For this review, take the finished solid that the model builds, in its own axes (mm). A direction names the side the tool comes from. Give positions to 0.01 mm unless a question says otherwise; leave off trailing zeros. Write each loop counter-clockwise with the first axis right and the second up, starting at its lowest first coordinate (ties: lowest second). Pieces come first, ordered by that corner, then holes. Notation, with made-up numbers: (7.25, 45.5) -> (11.25, 45.5) arc R18 ccw to (11.25, 57.5) -> close; hole circle Ø10 at (76, 66). An arc over 180 degrees is marked (long way). Return JSON: item names as keys, results as strings.
from build123d import *

# Parameters (mm, degrees)
SKIZZE1_W                                            = 40
SKIZZE1_H                                            = 7
AUFSATZ_LINEAR_AUSTRAGEN1_DEPTH                      = 35
SKIZZE2_W                                            = 12
SKIZZE2_H                                            = 6.1
SKIZZE2_R                                            = 0.6
AUFSATZ_LINEAR_AUSTRAGEN2_DEPTH                      = 14
FORMSENKUNG_F_R_M3_SENKSCHRAUBE_MIT_SCHL_D           = 3.4
FORMSENKUNG_F_R_M3_SENKSCHRAUBE_MIT_SCHL_CSINK_D     = 6.3
FORMSENKUNG_F_R_M3_SENKSCHRAUBE_MIT_SCHL_CSINK_ANGLE = 90
VERRUNDUNG1_R                                        = 3.5
SCHNITT_LINEAR_AUSTRAGEN1_DEPTH                      = 45.648628198
SCHNITT_LINEAR_AUSTRAGEN2_DEPTH                      = 2


with BuildPart() as part:
    # Skizze1 → Aufsatz-Linear austragen1 (new body)
    with BuildSketch(Plane(origin=(0, 0, 0), x_dir=(1, 0, 0), z_dir=(0, 1, 0))):
        with Locations((1.5, 0)):
            Rectangle(SKIZZE1_W, SKIZZE1_H)
    extrude(amount=AUFSATZ_LINEAR_AUSTRAGEN1_DEPTH)

    # Skizze2 → Aufsatz-Linear austragen2 (add)
    # profile 1 of 2: a face of its own
    with BuildSketch(Plane(origin=(0, 0, -3.5), x_dir=(-1, 0, 0), z_dir=(0, 0, -1))):
        with Locations((-15.5, 31.95)):
            Rectangle(SKIZZE2_W, SKIZZE2_H)
        with Locations((-15.5, 31.75)):
            Circle(SKIZZE2_R, mode=Mode.SUBTRACT)
    # profile 2 of 2: a face of its own
    with BuildSketch(Plane(origin=(0, 0, -3.5), x_dir=(-1, 0, 0), z_dir=(0, 0, -1))):
        with Locations((-15.5, 3.05)):
            Rectangle(SKIZZE2_W, SKIZZE2_H)
        with Locations((-15.5, 3.25)):
            Circle(SKIZZE2_R, mode=Mode.SUBTRACT)
    extrude(amount=AUFSATZ_LINEAR_AUSTRAGEN2_DEPTH)

    # Formsenkung für M3 Senkschraube mit Schlitz/Kreuzschlitz1 (through all)
    with Locations(Plane(origin=(0, 0, -3.5), x_dir=(-1, 0, 0), z_dir=(0, 0, -1))):
        with Locations((-5, 20), (5, 20), (5, 5), (-5, 5)):
            CounterSinkHole(FORMSENKUNG_F_R_M3_SENKSCHRAUBE_MIT_SCHL_D / 2, FORMSENKUNG_F_R_M3_SENKSCHRAUBE_MIT_SCHL_CSINK_D / 2, counter_sink_angle=FORMSENKUNG_F_R_M3_SENKSCHRAUBE_MIT_SCHL_CSINK_ANGLE)

    # Verrundung1
    verrundung1_edges = [part.edges().sort_by_distance(p)[0] for p in [
        (21.5, 17.5, 3.5),
        (-18.5, 17.5, 3.5),
        (-18.5, 17.5, -3.5),
    ]]
    fillet(verrundung1_edges, radius=VERRUNDUNG1_R - 0.0001)  # a hair under: the kernel refuses the full size

    # Skizze1<5> → Schnitt-Linear austragen1 (cut, through all)
    with BuildSketch(Plane(origin=(0, 0, 0), x_dir=(1, 0, 0), z_dir=(0, 1, 0))):
        with BuildLine():
            ThreePointArc((13.45, 0), (15, -1.55), (16.55, 0))
            Line((16.55, 0), (13.45, 0))
        make_face()
        with BuildLine():
            Line((13.45, 0), (16.55, 0))
            ThreePointArc((16.55, 0), (15, 1.55), (13.45, 0))
        make_face()
        with BuildLine():
            ThreePointArc((-16.55, 0), (-15, -1.55), (-13.45, 0))
            Line((-13.45, 0), (-16.55, 0))
        make_face()
        with BuildLine():
            Line((-16.55, 0), (-13.45, 0))
            ThreePointArc((-13.45, 0), (-15, 1.55), (-16.55, 0))
        make_face()
    extrude(amount=SCHNITT_LINEAR_AUSTRAGEN1_DEPTH, mode=Mode.SUBTRACT)

    # Skizze1<7> → Schnitt-Linear austragen2 (cut)
    with BuildSketch(Plane(origin=(0, 0, 0), x_dir=(1, 0, 0), z_dir=(0, 1, 0))):
        with BuildLine():
            ThreePointArc((-2.4, 0), (0, -2.4), (2.4, 0))
            Line((2.4, 0), (-2.4, 0))
        make_face()
        with BuildLine():
            Line((-2.4, 0), (2.4, 0))
            ThreePointArc((2.4, 0), (0, 2.4), (-2.4, 0))
        make_face()
    extrude(amount=SCHNITT_LINEAR_AUSTRAGEN2_DEPTH, mode=Mode.SUBTRACT)


solid = part.part
1. Add section A-A, the plane y = 20. Count the separate pieces of the cut face and the enclosed holes in it, plus the area to 3 significant figures.
Results found:
{"separate pieces": "3", "enclosed holes": "2", "area": "205 mm²"}
2. The part is to be moulded in two halves that separate along Z. For faces 1 (the cylindrical face through (13.45, 17.26, -0.07)), 2 (the cylindrical face through (5.8, 3.5, 0.8)), 3 (the cylindrical face through (-17.5, 17.74, 2.45)), 4 (the flat face through (15.5, 3.2, -3.5)), say which applies: +Z half, -Z half, draft (parallel to the pull), parting line (faces both ways), or undercut.
Results found:
{"face 1": "undercut", "face 2": "draft", "face 3": "+Z half", "face 4": "-Z half"}
3. Add section B-B, the plane x = -5. State the section outline as (y, z) points.
Results found:
{"outline": "(0, -3.5) -> (1.85, -3.5) -> (3.3, -2.05) -> (3.3, 3.5) -> (0, 3.5) -> close; (6.7, -2.05) -> (8.15, -3.5) -> (16.85, -3.5) -> (18.3, -2.05) -> (18.3, 3.5) -> (6.7, 3.5) -> close; (21.7, -2.05) -> (23.15, -3.5) -> (35, -3.5) -> (35, 3.5) -> (21.7, 3.5) -> close"}
4. For pin 1 (3 mm diameter, centred on y = 32, z = -14, fed in from -X); pin 2 (2.5 mm diameter, centred on x = 5, y = 20, fed in from -Z) (3 decimals); pin 3 (4 mm diameter, centred on x = -5, y = 20, fed in from -Z); pin 4 (1 mm diameter, centred on x = 15.5, y = 31.75, fed in from -Z), all flat-tipped, find the tip position at first contact; note any pin that passes through.
Results found:
{"pin 1": "stops at x = 9.5", "pin 2": "passes through", "pin 3": "stops at z = -2.35", "pin 4": "stops at z = -3.5"}
5. Add section C-C, the plane z = -9. State the section outline as (x, y) points.
Results found:
{"outline": "(9.5, 0) -> (21.5, 0) -> (21.5, 6.1) -> (9.5, 6.1) -> close; (9.5, 28.9) -> (21.5, 28.9) -> (21.5, 35) -> (9.5, 35) -> close; hole circle Ø1.2 at (15.5, 3.25); hole circle Ø1.2 at (15.5, 31.75)"}
6. For faces 5 (the flat face through (0, 2, 0)), 6 (the cylindrical face through (15.578, 32.345, -10.402)), 7 (the flat face through (9.5, 32, -10)), list the 3-axis set-ups (+Z, -Z, +X, -X, +Y, -Y) from which the entire face can be reached by the end or side of a thin tool; tool diameter is ignored.
Results found:
{"face 5": "-Y", "face 6": "-Z", "face 7": "-Z, -X, +Y, -Y"}
7. To check wall thickness, follow probe 1 along Y at (x, z) = (-5, -0.65); probe 2 along Y at (x, z) = (15.5, -5.75); probe 3 along X at (y, z) = (5, 0). State the ranges of each line that lie inside material, in increasing order.
Results found:
{"probe 1": "y = 0 to 3.3, 6.7 to 18.3, 21.7 to 35", "probe 2": "y = 0 to 2.65, 3.85 to 6.1, 28.9 to 31.15, 32.35 to 35", "probe 3": "x = -18.5 to -16.55, -13.45 to -6.7, -3.3 to 3.3, 6.7 to 13.45, 16.55 to 21.5"}
